Read the model definition and answer for the solid it produces. Units are mm, in the model's axes. A direction names the side the tool comes from. Round coordinates to 2 decimals unless told otherwise and drop trailing zeros. Loops run counter-clockwise (first coordinate to the right, second up) from the corner with the lowest first, then second, coordinate; pieces in that order, holes last. Notation, with made-up numbers: (-7, 50) - (37, 50) arc R30 cw to (37, 80) - close; hole circle Ø9 at (0, 22.5). An arc over 180 degrees is marked (long way). Answer as CSV lines item,"result".
```python
from build123d import *

# Parameters (mm, degrees)
F1_DEPTH = 25.4
F2_R     = 5.08


with BuildPart() as f1:
    # F0 (on Top) → F1 (new body)
    with BuildSketch(Plane.XY):
        Polygon((49.520503, 0), (0, 0), (0, 14.2875), (49.520503, 14.2875), (49.520503, 26.9875), (-77.479497, 26.9875), (-77.479497, 39.6875), (-90.179497, 39.6875), (-90.179497, 14.2875), (-26.679497, 14.2875), (-26.679497, -12.7), (49.520503, -12.7), align=None)
    extrude(amount=F1_DEPTH)

    # F2
    f2_edges = [f1.edges().sort_by_distance(p)[0] for p in [
        (49.520503, 14.2875, 12.7),
        (49.520503, 26.9875, 12.7),
        (49.520503, 20.6375, 0),
        (49.520503, 20.6375, 25.4),
        (49.520503, -12.7, 12.7),
        (49.520503, 0, 12.7),
        (49.520503, -6.35, 0),
        (49.520503, -6.35, 25.4),
        (-13.979497, 26.9875, 25.4),
        (-58.429497, 14.2875, 25.4),
        (-77.479497, 33.3375, 25.4),
        (-77.479497, 33.3375, 0),
        (-13.979497, 26.9875, 0),
        (-77.479497, 39.6875, 12.7),
        (-90.179497, 39.6875, 12.7),
        (-90.179497, 14.2875, 12.7),
        (-90.179497, 26.9875, 0),
        (-90.179497, 26.9875, 25.4),
        (-26.679497, -12.7, 12.7),
    ]]
    fillet(f2_edges, radius=F2_R)


solid = f1.part
```
1) A cutting plane is placed at B-B, the plane z = 7.5. Determine the outline of the cut face in (x, y), plus the area to 3 significant figures.
Entries:
outline,"(-90.18, 19.37) arc R5.08 ccw to (-85.1, 14.29) - (-26.68, 14.29) - (-26.68, -7.62) arc R5.08 ccw to (-21.6, -12.7) - (44.44, -12.7) arc R5.08 ccw to (49.52, -7.62) - (49.52, -5.08) arc R5.08 ccw to (44.44, 0) - (0, 0) - (0, 14.29) - (44.44, 14.29) arc R5.08 ccw to (49.52, 19.37) - (49.52, 21.91) arc R5.08 ccw to (44.44, 26.99) - (-77.48, 26.99) - (-77.48, 34.61) arc R5.08 ccw to (-82.56, 39.69) - (-85.1, 39.69) arc R5.08 ccw to (-90.18, 34.61) - close"
area,"3,240 mm^2"
2) A cutting plane is placed at C-C, the plane x = -63. Determine the outline of the cut face in (y, z), plus the area to 3 significant figures.
Entries:
outline,"(14.29, 0) - (21.91, 0) arc R5.08 ccw to (26.99, 5.08) - (26.99, 20.32) arc R5.08 ccw to (21.91, 25.4) - (19.37, 25.4) arc R5.08 ccw to (14.29, 20.32) - close"
area,"306 mm^2"
3) Each of these flat-tipped pins is pushed along its axis until it touches: P1, Ø12, axis at x = 1.5, z = 16, coming from the +Y side; P2, Ø1, axis at y = 5, z = 21.5, coming from the -X side; P3, Ø3, axis at y = 25, z = 11, coming from the +X side. Where does it stop, or does it pass through?
Entries:
P1,"stops at y = 26.99"
P2,"stops at x = -26.68"
P3,"stops at x = 49.26"
4) A tool of negligible diameter and unlimited length cuts with its end or side. For faces 1 (the face through (47.993, -1.449, 12.878)), 2 (the face through (-77.479, 31, 13)), 3 (the face through (-19.95, 25.54, 23.87)), 4 (the face through (-19.95, 25.54, 1.53)), 5 (the face through (-56, 14.288, 10)), from which of +Z, -Z, +X, -X, +Y, -Y can it reach the whole face along a straight path? Write none if from no direction.
Entries:
face 1,"+Z, -Z, +X"
face 2,"+Z, -Z, +X, +Y"
face 3,"+Z, +X, +Y"
face 4,"-Z, +X, +Y"
face 5,"+Z, -Z, -X, -Y"
5) Find the intervals of material crossed by line 1 (Y direction, x = 25.5, z = 20.75); line 2 (X direction, y = 9, z = 11.5); line 3 (Y direction, x = -58, z = 15.5), in increasing order.
Entries:
line 1,"y = -12.7 to 0, 14.29 to 26.97"
line 2,"x = -26.68 to 0"
line 3,"y = 14.29 to 26.99"
6) A cutting plane is placed at D-D, the plane y = 1.5. Determine the outline of the cut face in (x, z), plus the area to 3 significant figures.
Entries:
outline,"(-26.68, 0) - (0, 0) - (0, 25.4) - (-26.68, 25.4) - close"
area,"678 mm^2"
7) A cutting plane is placed at A-A, the plane x = 16. Determine the outline of the cut face in (y, z).
Entries:
outline,"(-12.7, 0) - (0, 0) - (0, 25.4) - (-12.7, 25.4) - close; (14.29, 0) - (21.91, 0) arc R5.08 ccw to (26.99, 5.08) - (26.99, 20.32) arc R5.08 ccw to (21.91, 25.4) - (14.29, 25.4) - close"
